Verification items for the finished model (mm, model axes). A direction names the side the tool comes from. Give positions to 0.01 mm unless a question says otherwise; leave off trailing zeros. Loops run counter-clockwise (first coordinate to the right, second up) from the corner with the lowest first, then second, coordinate; pieces in that order, holes last. Notation, with made-up numbers: (67, 34) - (97, 34) arc R30 ccw to (97, 59) - close; hole circle Ø10 at (2.25, -18.5). An arc over 180 degrees is marked (long way). Answer in a Markdown table with one row per item.
```python
from build123d import *

# Parameters (mm, degrees)
F1_DEPTH  = 50
F3_DEPTH  = 10
F5_R      = 3.75
F6_DEPTH  = 10.001
F4_R      = 3.75
F7_DEPTH  = 30.001
F9_DEPTH  = 5
F11_DEPTH = 5
F13_DEPTH = 10


with BuildPart() as f1:
    # F0 (on Top) → F1 (new body)
    with BuildSketch(Plane.XY):
        Polygon((0, 40), (0, 0), (10, 0), (10, 35.8578643763), (35.3553390593, 61.2132034356), (28.2842712475, 68.2842712475), align=None)
    extrude(amount=F1_DEPTH)

    # F2 (on face) → F3 (join)
    with BuildSketch(Plane.XY.offset(50)):
        Polygon((86.5685424949, 10), (35.3553390593, 61.2132034356), (10, 35.8578643763), (10, 0), (125, 0), (125, 10), align=None)
        Polygon((35.3553390593, 47.0710678119), (72.4264068712, 10), (20, 10), (20, 31.7157287525), align=None, mode=Mode.SUBTRACT)
    extrude(amount=-F3_DEPTH)

    # F5 (on face) → F6 (cut, through all)
    with BuildSketch(Plane.YZ.offset(10)):
        with Locations((17.9289321881, 20)):
            Circle(F5_R)
    extrude(amount=-F6_DEPTH, mode=Mode.SUBTRACT)

    # F4 (on face) → F7 (cut, through all)
    with BuildSketch(Plane(origin=(-12.9289321881, 12.9289321881, 0), x_dir=(0.7071067812, 0.7071067812, 0), z_dir=(0.7071067812, -0.7071067812, 0))):
        with Locations((50.3553390593, 20)):
            Circle(F4_R)
    extrude(amount=-F7_DEPTH, mode=Mode.SUBTRACT)

    # F8 (on face) → F9 (join)
    with BuildSketch(Plane.XZ):
        Polygon((10, 14.1421356237), (10, 0), (50, 40), (35.8578643763, 40), align=None)
    extrude(amount=-F9_DEPTH)

    # F10 (on face) → F11 (join)
    with BuildSketch(Plane(origin=(48.2842712475, 48.2842712475, 0), x_dir=(-0.7071067812, 0.7071067812, 0), z_dir=(0.7071067812, 0.7071067812, 0))):
        Polygon((-21.7157287525, 40), (18.2842712475, 0), (18.2842712475, 14.1421356237), (-7.5735931288, 40), align=None)
    extrude(amount=-F11_DEPTH)

    # F12 (on face) → F13 (join, through all)
    with BuildSketch(Plane.XY.offset(50)):
        Polygon((14.1421356237, 0), (0, 0), (86.5685424949, -86.5685424949), (125, -86.5685424949), (125, -76.5685424949), (125, 0), (115, 0), (100.8578643763, 0), (57.5, -43.3578643763), align=None)
        Polygon((64.5710678119, -50.4289321881), (115, 0), (115, -76.5685424949), (90.7106781187, -76.5685424949), align=None, mode=Mode.SUBTRACT)
        Polygon((115, -76.5685424949), (115, 0), (64.5710678119, -50.4289321881), (90.7106781187, -76.5685424949), align=None)
    extrude(amount=-F13_DEPTH)


solid = f1.part
```
Q1. Sectioned sample at B-B (z = 44). Record the cut outline in (x, y), and give its area (3 significant figures).
Completed:
| item | result |
|---|---|
| outline | (0, 0) - (86.57, -86.57) - (125, -86.57) - (125, 10) - (86.57, 10) - (28.28, 68.28) - (0, 40) - close; hole (14.14, 0) - (57.5, -43.36) - (100.86, 0) - close; hole (20, 10) - (72.43, 10) - (35.36, 47.07) - (20, 31.72) - close |
| area | 8,250 mm^2 |
Q2. Sectioned sample at A-A (z = 26). Record the cut outline in (x, y).
Completed:
| item | result |
|---|---|
| outline | (0, 0) - (10, 0) - (10, 35.86) - (35.36, 61.21) - (28.28, 68.28) - (0, 40) - close; (21.86, 0) - (36, 0) - (36, 5) - (21.86, 5) - close; (40.2, 49.29) - (50.2, 39.29) - (53.74, 42.83) - (43.74, 52.83) - close |
Q3. Sectioned sample at C-C (y = -39). Record the cut outline in (x, z).
Completed:
| item | result |
|---|---|
| outline | (39, 40) - (53.14, 40) - (53.14, 50) - (39, 50) - close; (61.86, 40) - (125, 40) - (125, 50) - (61.86, 50) - close |
Q4. Draft check along X on faces 1 (the face through (23.11, 2.46, 27.25)), 2 (the face through (47.95, 45.13, 20.28)), 3 (the face through (25, 5, 25)), 4 (the face through (27.57, 39.286, 45.07)). Enter one of: +X half, -X half, draft (parallel to the pull), parting line (faces both ways), or undercut.
Completed:
| item | result |
|---|---|
| face 1 | undercut |
| face 2 | +X half |
| face 3 | draft |
| face 4 | undercut |
Q5. Sectioned sample at D-D (x = 44.5). Record the cut outline in (y, z).
Completed:
| item | result |
|---|---|
| outline | (-44.5, 40) - (-30.36, 40) - (-30.36, 50) - (-44.5, 50) - close; (0, 34.5) - (5, 34.5) - (5, 40) - (10, 40) - (10, 50) - (0, 50) - close; (37.93, 40) - (52.07, 40) - (52.07, 50) - (37.93, 50) - close; (45, 17.93) - (52.07, 12.93) - (52.07, 27.07) - (45, 32.07) - close |
Q6. Tool access check on faces 5 (the face through (20, 21, 45)), 6 (the face through (30, 2, 20)), 7 (the face through (39, 0, 31)), 8 (the face through (106, 10, 45)), 9 (the face through (125, -39, 45)). Record the directions out of +Z, -Z, +X, -X, +Y, -Y that give a thin tool (end or side, any length) a straight path to the whole face; none if there is none.
Completed:
| item | result |
|---|---|
| face 5 | +Z, -Z |
| face 6 | -Z, +X, -Y |
| face 7 | -Z |
| face 8 | +Z, -Z, +X, +Y |
| face 9 | +Z, -Z, +X, +Y, -Y |
Q7. Go/stop test with flat-tipped pins: P1, Ø20, axis at x = 38.5, z = 24, coming from the +Y side; P2, Ø8, axis at x = 47.5, z = 44.5, coming from the +Y side; P3, Ø5, axis at y = 16, z = 47, coming from the +X side; P4, Ø8, axis at x = 21, y = 28.5, coming from the +Z side. Record where each tip stops, or that it passes through.
Completed:
| item | result |
|---|---|
| P1 | y = 68.07 |
| P2 | y = 53.07 |
| P3 | x = 83.07 |
| P4 | z = 50 |
Q8. Thickness scan on line 1 (X direction, y = -35, z = 42); line 2 (X direction, y = 42.5, z = 24); line 3 (X direction, y = 6, z = 36). Record the ranges inside material, lowest first.
Completed:
| item | result |
|---|---|
| line 1 | 35 to 49.14, 65.86 to 125 |
| line 2 | 2.5 to 16.64, 47 to 50.58 |
| line 3 | 0 to 10 |
